For this review, take the finished solid that the model builds, in its own axes (mm). Face numbers are marked on the shaded views. A direction names the side the tool comes from. Round coordinates to 2 decimals unless told otherwise and drop trailing zeros. Order: outer loops, then holes, each group sorted by start corner. A loop starts at its lowest first (then second) coordinate and runs counter-clockwise, first axis right, second up. Notation, with made-up numbers: M 22.5,46 L 55.5,46 A28 ccw 55.5,80 Z; hole C 23,76 d7. An arc over 180 degrees is marked long. Write item = value, one per line. Start each with the question number.
from build123d import *

# Parameters (mm, degrees)
EXTRUDE_1_DEPTH        = 10
CUT_EXTRUDE_1_DEPTH    = 5
FILLET_1_R             = 2
HOLE_WIZARD_M4_1_D     = 3.3
HOLE_WIZARD_M4_1_DEPTH = 6
HOLE_WIZARD_M4_2_D     = 3.3
FILLET_2_R             = 2
SKETCH_23_R            = 4
CUT_EXTRUDE_3_DEPTH    = 1


with BuildPart() as part:
    # 草图1 → 凸台-拉伸1 (new body)
    with BuildSketch(Plane.XY):
        Polygon((0, 0), (0, 6), (-20, 6), (-20, 12.5), (0, 12.5), (0, 18.5), (-20, 18.5), (-11.634836963, 49.719213469), (-21.294095226, 52.30740392), (-30.352761804, 18.5), (-30.352761804, 0), align=None)
    extrude(amount=EXTRUDE_1_DEPTH)

    # 草图2 → 切除-拉伸1 (cut)
    with BuildSketch(Plane.XY.offset(10)):
        Polygon((-21.294095226, 52.30740392), (-11.634836963, 49.719213469), (-14.223027414, 40.059955206), (-23.882285677, 42.648145657), align=None)
    extrude(amount=-CUT_EXTRUDE_1_DEPTH, mode=Mode.SUBTRACT)

    # 圆角1
    fillet_1_edges = [part.edges().sort_by_distance(p)[0] for p in [
        (-20, 18.5, 5),
    ]]
    fillet(fillet_1_edges, radius=FILLET_1_R)

    # M4 螺纹孔1
    with Locations(Plane(origin=(0, 18.5, 0), x_dir=(1, 0, 0), z_dir=(0, 1, 0))):
        with Locations((-10, -5)):
            Hole(HOLE_WIZARD_M4_1_D / 2, depth=HOLE_WIZARD_M4_1_DEPTH)

    # M4 螺纹孔2 (through all)
    with Locations(Plane.XY.offset(5)):
        with Locations((-17.75856132, 46.183679563)):
            Hole(HOLE_WIZARD_M4_2_D / 2)

    # 圆角2
    fillet_2_edges = [part.edges().sort_by_distance(p)[0] for p in [
        (-30.352761804, 0, 5),
    ]]
    fillet(fillet_2_edges, radius=FILLET_2_R)

    # 草图23 → 切除-拉伸3 (cut)
    with BuildSketch(Plane(origin=(0, 0, 0), x_dir=(-1, 0, 0), z_dir=(0, 0, -1))):
        with Locations((17.75856132, 46.183679563)):
            Circle(SKETCH_23_R)
    extrude(amount=-CUT_EXTRUDE_3_DEPTH, mode=Mode.SUBTRACT)


solid = part.part
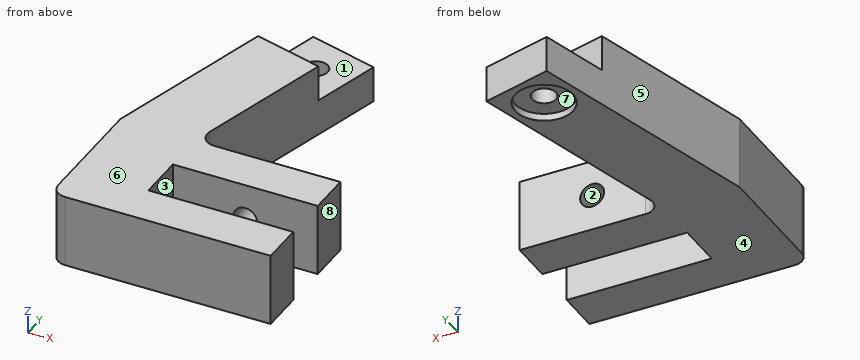
(1) For the marked faces 1, 2, 3 and 4, list the 3-axis set-ups (+Z, -Z, +X, -X, +Y, -Y) from which the entire face can be reached by the end or side of a thin tool; tool diameter is ignored.
(2) We need section C-C, the plane x = -10. Write out the cut boundary in (y, z).
(3) Insertion check: pin 1 (5 mm diameter, centred on x = -7, z = 7.5, fed in from +Y); pin 2 (2 mm diameter, centred on x = -12, z = 4, fed in from +Y) (3 decimals); pin 3 (2.5 mm diameter, centred on x = -10, z = 5, fed in from +Y). Each pin has a flat end and moves straight along its axis. Give the tip position at first contact, or say it passes through.
(4) We need section B-B, the plane z = 8.75. Write out the cut boundary in (x, y), then the cut area to 3 significant figures.
(5) We need section D-D, the plane x = -15. Write out the cut boundary in (y, z).
(6) Draft analysis for pull direction X (two halves, no side actions). For the marked faces 5, 6, 7 and 8, state which applies: released by +X, released by -X, zero draft, split by the parting line, or undercut.
(7) We need section A-A, the plane y = 17. Write out the cut boundary in (x, z).
(8) For line 1 along Y through (x, z) = (-13, 7.75); line 2 along X through (y, z) = (13.85, 5); line 3 along Z through (x, y) = (-10, 16), list the stretches that pass through material, from the lowest coordinate up.
Values:
q1.face_1 = +Z, +X, +Y
q1.face_2 = +Y
q1.face_3 = +Z, -Z, +X
q1.face_4 = -Z, +X, -X, +Y, -Y
q2.outline = M 0,0 L 6,0 L 6,10 L 0,10 Z; M 12.5,0 L 18.5,0 L 18.5,3.35 L 12.5,3.35 Z; M 12.5,6.65 L 18.5,6.65 L 18.5,10 L 12.5,10 Z
q3.pin_1 = 18.5
q3.pin_2 = 50.085
q3.pin_3 = 6
q4.outline = M -30.35,2 A2 ccw -28.35,0 L 0,0 L 0,6 L -20,6 L -20,12.5 L 0,12.5 L 0,18.5 L -17.39,18.5 A2 cw -19.33,21.02 L -14.22,40.06 L -23.88,42.65 L -30.35,18.5 Z
q4.area = 669 mm²
q5.outline = M 0,0 L 6,0 L 6,10 L 0,10 Z; M 12.5,0 L 18.5,0 L 18.5,10 L 12.5,10 Z; M 37.16,0 L 43.29,0 L 43.29,1 L 49.08,1 L 49.08,0 L 50.62,0 L 50.62,5 L 40.27,5 L 40.27,10 L 37.16,10 Z
q6.face_5 = released by -X
q6.face_6 = zero draft
q6.face_7 = undercut
q6.face_8 = released by +X
q7.outline = M -30.35,0 L 0,0 L 0,10 L -30.35,10 Z; hole C -10,5 d3.3
q8.line_1 = 0 to 6, 12.5 to 18.5
q8.line_2 = -30.35 to -11.65, -8.35 to 0
q8.line_3 = 0 to 3.35, 6.65 to 10
